```python
from build123d import *

# Parameters (mm, degrees)
F1_DEPTH = 3


with BuildPart() as f1:
    # F0 (on Top) → F1 (new body)
    with BuildSketch(Plane.XY):
        with BuildLine():
            Line((22.9510348351, 1.5), (24.9549594269, 1.5))
            ThreePointArc((24.9549594269, 1.5), (0, 25), (-24.9549594269, 1.5))
            Line((-24.9549594269, 1.5), (-22.9510348351, 1.5))
            ThreePointArc((-22.9510348351, 1.5), (0, 23), (22.9510348351, 1.5))
        make_face()
        with BuildLine():
            Line((-22.9510348351, 1.5), (-24.9549594269, 1.5))
            ThreePointArc((-24.9549594269, 1.5), (-25, 0), (-24.9549594269, -1.5))
            Line((-24.9549594269, -1.5), (-22.9510348351, -1.5))
            ThreePointArc((-22.9510348351, -1.5), (-23, 0), (-22.9510348351, 1.5))
        make_face()
        with BuildLine():
            ThreePointArc((-24.9549594269, -1.5), (0, -25), (24.9549594269, -1.5))
            Line((24.9549594269, -1.5), (22.9510348351, -1.5))
            ThreePointArc((22.9510348351, -1.5), (0, -23), (-22.9510348351, -1.5))
            Line((-22.9510348351, -1.5), (-24.9549594269, -1.5))
        make_face()
        with BuildLine():
            ThreePointArc((24.9549594269, -1.5), (24.9887373198, -0.7503380327), (25, 0))
            ThreePointArc((25, 0), (24.9887373198, 0.7503380327), (24.9549594269, 1.5))
            Line((24.9549594269, 1.5), (22.9510348351, 1.5))
            ThreePointArc((22.9510348351, 1.5), (22.9877554494, 0.7503994915), (23, 0))
            ThreePointArc((23, 0), (22.9877554494, -0.7503994915), (22.9510348351, -1.5))
            Line((22.9510348351, -1.5), (24.9549594269, -1.5))
        make_face()
        with BuildLine():
            ThreePointArc((24.9549594269, 1.5), (24.9887373198, 0.7503380327), (25, 0))
            ThreePointArc((25, 0), (24.9887373198, -0.7503380327), (24.9549594269, -1.5))
            Line((24.9549594269, -1.5), (27.5, -1.5))
            Line((27.5, -1.5), (27.5, 1.5))
            Line((27.5, 1.5), (24.9549594269, 1.5))
        make_face()
        with BuildLine():
            ThreePointArc((-24.9549594269, -1.5), (-25, 0), (-24.9549594269, 1.5))
            Line((-24.9549594269, 1.5), (-27.5, 1.5))
            Line((-27.5, 1.5), (-27.5, -1.5))
            Line((-27.5, -1.5), (-24.9549594269, -1.5))
        make_face()
    extrude(amount=F1_DEPTH)


solid = f1.part
```
Geometry check sheet. Reference: the model listing, model coordinates, mm. A direction names the side the tool comes from. Round coordinates to 2 decimals unless told otherwise and drop trailing zeros. Loops run counter-clockwise (first coordinate to the right, second up) from the corner with the lowest first, then second, coordinate; pieces in that order, holes last. Notation, with made-up numbers: M 71.5,53 L 102.5,53 A12 cw 102.5,60 Z; hole C -37,57 d8. An arc over 180 degrees is marked long. Return JSON: item names as keys, results as strings. Group by question number.
(1) Set-up check for faces 1 (the face through (-26, -1.5, 1)), 2 (the face through (26, -1.5, 1)), 3 (the face through (16, 17, 0)), 4 (the face through (26, 1.5, 1)), 5 (the face through (-26, 1.5, 1)): record each of +Z, -Z, +X, -X, +Y, -Y from which the full face is reachable in a straight line by a thin tool's end or side.
(2) Section check A-A, the plane x = 0. Enter the section's corners in (y, z).
(3) Go/stop test with flat-tipped pins: pin 1 (2 mm diameter, centred on x = -14, y = -16, fed in from -Z); pin 2 (1 mm diameter, centred on x = -5.5, z = 2.5, fed in from -Y); pin 3 (1.3 mm diameter, centred on x = 26, z = 1, fed in from -Y). Record where each tip stops, or that it passes through.
(4) Scan lines: line 1 along X through (y, z) = (3, 0.45); line 2 along Y through (x, z) = (18, 2.35); line 3 along X through (y, z) = (-11.5, 2.5). Record each from-to range of solid material in increasing order. Write a range as [from, to].
(5) Section check C-C, the plane y = -6.5. Enter the section's corners in (x, z).
Data:
{
 "1": {"face 1": "+Z, -Z, -X, -Y", "face 2": "+Z, -Z, +X, -Y", "face 3": "-Z, +X, -X, +Y, -Y", "face 4": "+Z, -Z, +X, +Y", "face 5": "+Z, -Z, -X, +Y"},
 "2": {"outline": "M -25,0 L -23,0 L -23,3 L -25,3 Z; M 23,0 L 25,0 L 25,3 L 23,3 Z"},
 "3": {"pin 1": "through", "pin 2": "y = -24.49", "pin 3": "y = -1.5"},
 "4": {"line 1": "[-24.82, -22.8], [22.8, 24.82]", "line 2": "[-17.35, -14.32], [14.32, 17.35]", "line 3": "[-22.2, -19.92], [19.92, 22.2]"},
 "5": {"outline": "M -24.14,0 L -22.06,0 L -22.06,3 L -24.14,3 Z; M 22.06,0 L 24.14,0 L 24.14,3 L 22.06,3 Z"}
}
